The listing builds one solid part. Answer for the finished solid, in the listing's coordinates (mm). A direction names the side the tool comes from. Round coordinates to 2 decimals unless told otherwise and drop trailing zeros. Order: outer loops, then holes, each group sorted by start corner. A loop starts at its lowest first (then second) coordinate and runs counter-clockwise, first axis right, second up. Notation, with made-up numbers: (20, -11) - (36, -11) arc R22 ccw to (36, 27) - close; hole circle Ø3 at (72, 50). An arc over 180 degrees is marked (long way). Use CSV: the item, a comma, the result in double quotes. Start each with the question number.
Item 1: Find section A-A, the plane x = 0. Give the vertices of the cut face in (y, z).
Item 2: Straight lines are drawn through the part: line 1 along Y through (x, z) = (0.2, -0.6); line 2 along X through (y, z) = (3, 0); line 3 along X through (y, z) = (8.25, -0.25). For each, find the intervals that lie inside material, in ascending order. Write a range as [from, to].
Item 3: Find section B-B, the plane z = 0. Give the vertices of the cut face in (x, y).
Item 4: For faces 1 (the cylindrical face through (-0.108, 4.93, 0.488)), 2 (the flat face through (0, -0.6, 0)), determine the directions among +Z, -Z, +X, -X, +Y, -Y from which every point of the face is accessible in a straight line to the end or side of a thin tool.
Item 5: Find section C-C, the plane y = 1.5. Give the vertices of the cut face in (x, z), plus the area to 3 significant figures.
```python
from build123d import *

# Parameters (mm, degrees)
SKETCH1_R           = 0.5
BOSS_EXTRUDE1_DEPTH = 10
SKETCH2_R           = 0.9
BOSS_EXTRUDE2_DEPTH = 0.6
FILLET1_R           = 0.3


with BuildPart() as part:
    # Sketch1 → Boss-Extrude1 (new body)
    with BuildSketch(Plane(origin=(0, 0, 0), x_dir=(1, 0, 0), z_dir=(0, 1, 0))):
        Circle(SKETCH1_R)
    extrude(amount=BOSS_EXTRUDE1_DEPTH)

    # Sketch2 → Boss-Extrude2 (add)
    with BuildSketch(Plane.XZ):
        Circle(SKETCH2_R)
    extrude(amount=BOSS_EXTRUDE2_DEPTH)

    # Fillet1
    fillet1_edges = [part.edges().sort_by_distance(p)[0] for p in [
        (-0.9, -0.6, 0),
    ]]
    fillet(fillet1_edges, radius=FILLET1_R)


solid = part.part
```
Worked out:
1,outline,"(-0.6, -0.6) arc R0.3 ccw to (-0.3, -0.9) - (0, -0.9) - (0, -0.5) - (10, -0.5) - (10, 0.5) - (0, 0.5) - (0, 0.9) - (-0.3, 0.9) arc R0.3 ccw to (-0.6, 0.6) - close"
2,line 1,"y = [-0.6, 0]"
2,line 2,"x = [-0.5, 0.5]"
2,line 3,"x = [-0.43, 0.43]"
3,outline,"(-0.9, -0.3) arc R0.3 ccw to (-0.6, -0.6) - (0.6, -0.6) arc R0.3 ccw to (0.9, -0.3) - (0.9, 0) - (0.5, 0) - (0.5, 10) - (-0.5, 10) - (-0.5, 0) - (-0.9, 0) - close"
4,face 1,"+Y"
4,face 2,"+Z, -Z, +X, -X, -Y"
5,outline,"circle Ø1 at (0, 0)"
5,area,"0.785 mm²"
